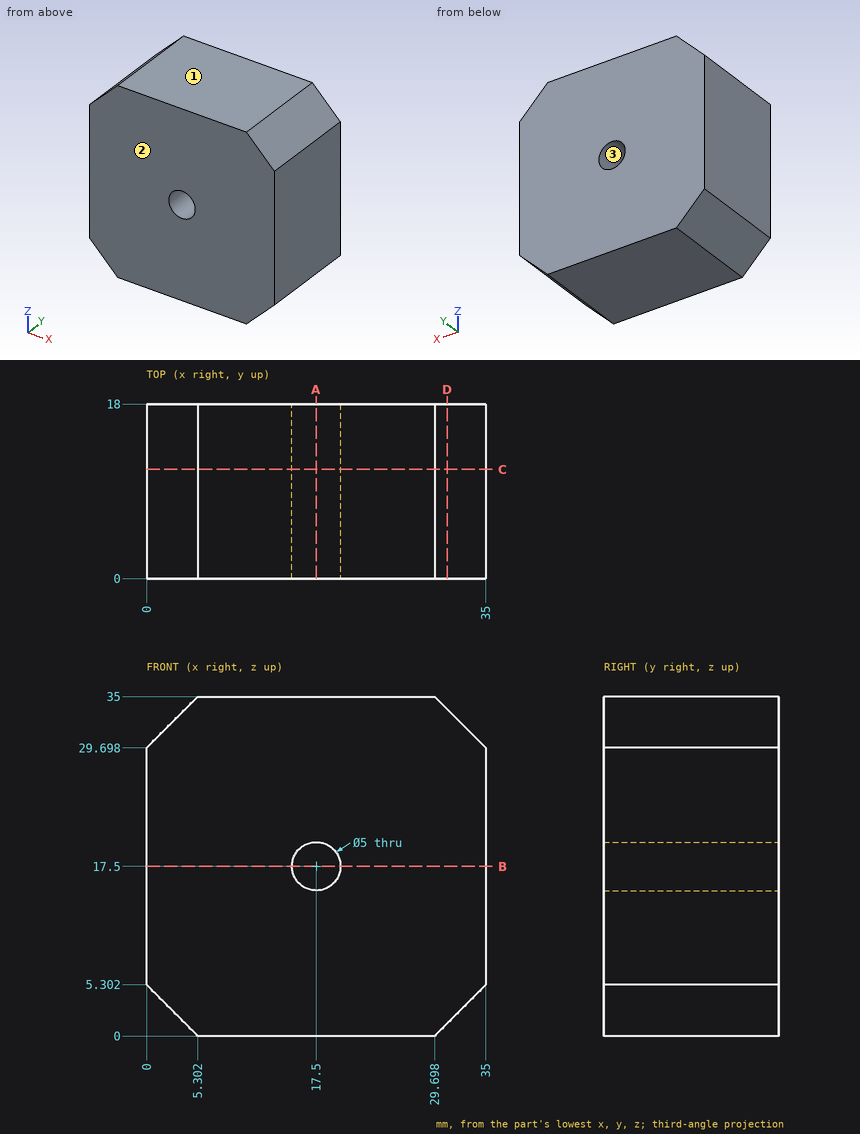
Could you check a few things on this drawing? It's one solid part, dimensions in mm from its lowest x, y, z. Coordinates: 2 decimals unless noted, no trailing zeros. Write each loop counter-clockwise with the first axis right and the second up, starting at its lowest first coordinate (ties: lowest second). Pieces come first, ordered by that corner, then holes. Notation, with made-up numbers: (-21.75, -8.75) - (-12.75, -8.75) arc R27 ccw to (-12.75, 7.25) - close; hole circle Ø1 at (62.5, 29). An arc over 180 degrees is marked (long way). Put each result on its own line as item: value. Start each with the question number.
Q1. I want a section at C-C on y = 11.25. Write out the boundary of the cut face in (x, z), plus the area to 3 significant figures.
Q2. I want a section at B-B on z = 17.5. Write out the boundary of the cut face in (x, y), plus the area to 3 significant figures.
Q3. I want a section at D-D on x = 31. Write out the boundary of the cut face in (y, z).
Q4. I'm going to push a flat-ended pin straight in: P1, Ø1, axis at y = 14, z = 31, coming from the +X side. Where does the tip first touch, or does it pass through?
Q5. Thinking about a two-plate mould opening in Z: for the marked faces 1, 2 and 3, which applies, pulls with the +Z half, pulls with the -Z half, needs draft (parallel to the pull), parting line crosses it, or undercut?
Q6. Please list where these lines run through material, in increasing order: L1, parallel to Z at x = 17.5, y = 12.5; L2, parallel to X at y = 1.25, z = 16.5.
Q7. I want a section at A-A on x = 17.5. Write out the boundary of the cut face in (y, z), plus the area to 3 significant figures.
Checks:
1. outline: (0, 5.3) - (5.3, 0) - (29.7, 0) - (35, 5.3) - (35, 29.7) - (29.7, 35) - (5.3, 35) - (0, 29.7) - close; hole circle Ø5 at (17.5, 17.5)
1. area: 1,150 mm²
2. outline: (0, 0) - (15, 0) - (15, 18) - (0, 18) - close; (20, 0) - (35, 0) - (35, 18) - (20, 18) - close
2. area: 540 mm²
3. outline: (0, 1.3) - (18, 1.3) - (18, 33.7) - (0, 33.7) - close
4. P1: x = 34.2
5. face 1: pulls with the +Z half
5. face 2: needs draft
5. face 3: undercut
6. L1: 0 to 15, 20 to 35
6. L2: 0 to 15.21, 19.79 to 35
7. outline: (0, 0) - (18, 0) - (18, 15) - (0, 15) - close; (0, 20) - (18, 20) - (18, 35) - (0, 35) - close
7. area: 540 mm²
